Source: CAD feature listing. Evaluate the final solid. Frame: model axes, mm. A direction names the side the tool comes from. Give positions to 0.01 mm unless a question says otherwise; leave off trailing zeros. Order: outer loops, then holes, each group sorted by start corner. A loop starts at its lowest first (then second) coordinate and runs counter-clockwise, first axis right, second up.
```python
from build123d import *

# Parameters (mm, degrees)
SKETCH1_W           = 25
SKETCH1_H           = 50
BOSS_EXTRUDE1_DEPTH = 30.875
CUT_EXTRUDE1_REACH  = 82.432


with BuildPart() as part:
    # Sketch1 → Boss-Extrude1 (new, symmetric)
    with BuildSketch(Plane.XY):
        with Locations((0, -25)):
            Rectangle(SKETCH1_W, SKETCH1_H)
    extrude(amount=BOSS_EXTRUDE1_DEPTH, both=True)

    # Sketch2 → Cut-Extrude1 (cut, up to next)
    with BuildSketch(Plane(origin=(0, 0, -30.875), x_dir=(-1, 0, 0), z_dir=(0, 0, -1)), mode=Mode.PRIVATE) as cut_extrude1_sk1:
        with BuildLine():
            Line((-2.363703305, -46.96472382), (-3.177003107, -50))
            Line((-3.177003107, -50), (6.177003107, -50))
            Line((6.177003107, -50), (5.363703305, -46.96472382))
            ThreePointArc((5.363703305, -46.96472382), (1.5, -44), (-2.363703305, -46.96472382))
        make_face()
    cut_extrude1_tool1 = extrude(cut_extrude1_sk1.sketch, amount=-CUT_EXTRUDE1_REACH, mode=Mode.PRIVATE) & part.part
    add(cut_extrude1_tool1.solids().sort_by_distance((-1.5, -47.423831, -30.875))[0], mode=Mode.SUBTRACT)


solid = part.part
```
1) Section query A-A, the plane z = -18.5. Return the cut outline in (x, y), and give its area (3 significant figures).
Report:
outline: (-12.5, -50) - (-6.18, -50) - (-5.36, -46.96) arc R4 cw to (2.36, -46.96) - (3.18, -50) - (12.5, -50) - (12.5, 0) - (-12.5, 0) - close
area: 1,210 mm2
2) Draft query along X for faces 1 (the flat face through (2.765, -48.461, -0.432)), 2 (the flat face through (-12.5, -25, 0)), 3 (the flat face through (0, 0, 0)). Return one class per face: +X half, -X half, draft (parallel to the pull), parting line (faces both ways), or undercut.
Report:
face 1: undercut
face 2: -X half
face 3: draft
3) Section query B-B, the plane y = -45. Return the cut outline in (x, z) (3 decimals).
Report:
outline: (-12.5, -30.875) - (-4.146, -30.875) - (-4.146, 30.875) - (-12.5, 30.875) - close; (1.146, -30.875) - (12.5, -30.875) - (12.5, 30.875) - (1.146, 30.875) - close
4) Pin query (flat end, axial travel): pin 1 (10 mm diameter, centred on x = 7, z = 8.5, fed in from +Y). Return the tip coordinate at first contact, or that it passes through.
Report:
pin 1: stops at y = 0
5) Material intervals for L1, parallel to Y at x = -0.75, z = 1; L2, parallel to Y at x = -3.5, z = -1, sorted ascending.
Report:
L1: y = -44.07 to 0
L2: y = -44.54 to 0
6) Reachability of faces 4 (the flat face through (0, -25, 30.875)), 5 (the flat face through (-5.776, -48.504, -0.432)) from +Z, -Z, +X, -X, +Y, -Y: full face, straight path, thin tool, end or side. Return the list, or none.
Report:
face 4: +Z, +X, -X, +Y, -Y
face 5: +Z, -Z, -Y
7) Section query C-C, the plane x = -1.5. Return the cut outline in (y, z) (3 decimals), and give its area (3 significant figures).
Report:
outline: (-44, -30.875) - (0, -30.875) - (0, 30.875) - (-44, 30.875) - close
area: 2,720 mm2
